```python
from build123d import *

# Parameters (mm, degrees)
SKETCH_1_W                      = 10
SKETCH_1_H                      = 110
CUT_EXTRUDE_1_REACH             = 12
SKETCH_2_R                      = 8.2
CUT_EXTRUDE_1_DIRECTION_2_DEPTH = 5
SKETCH_3_R                      = 1.4
CUT_EXTRUDE_2_DEPTH             = 11.0000001
CUT_EXTRUDE_2_DEPTH_BACK        = 11.0000001
FILLET_1_R                      = 10
FILLET_2_R                      = 10


with BuildPart() as part:
    # Sketch 1 → Revolve 1 (revolve)
    with BuildSketch(Plane.XY):
        with Locations((5, 55)):
            Rectangle(SKETCH_1_W, SKETCH_1_H)
    revolve(axis=Axis((0, 0, 0), (0, 1, 0)))

    # Sketch 2 → Cut-Extrude 1 (cut, up to next)
    with BuildSketch(Plane.XY, mode=Mode.PRIVATE) as cut_extrude_1_sk1:
        with Locations((0, 30)):
            Circle(SKETCH_2_R)
    cut_extrude_1_tool1 = extrude(cut_extrude_1_sk1.sketch, amount=-CUT_EXTRUDE_1_REACH, mode=Mode.PRIVATE) & part.part
    add(cut_extrude_1_tool1.solids().sort_by_distance((0, 30, 0))[0], mode=Mode.SUBTRACT)

    # Sketch 2 → Cut-Extrude 1 direction 2 (cut)
    with BuildSketch(Plane.XY):
        with Locations((0, 30)):
            Circle(SKETCH_2_R)
    extrude(amount=CUT_EXTRUDE_1_DIRECTION_2_DEPTH, mode=Mode.SUBTRACT)

    # Sketch 3 → Cut-Extrude 2 (cut, two sides)
    with BuildSketch(Plane(origin=(0, 0, 0), x_dir=(0, 0, -1), z_dir=(1, 0, 0))) as cut_extrude_2_sk:
        with Locations((0, 30)):
            Circle(SKETCH_3_R)
    extrude(amount=CUT_EXTRUDE_2_DEPTH, mode=Mode.SUBTRACT)
    extrude(cut_extrude_2_sk.sketch, amount=-CUT_EXTRUDE_2_DEPTH_BACK, mode=Mode.SUBTRACT)

    # Fillet 1
    fillet_1_edges = [part.edges().sort_by_distance(p)[0] for p in [
        (-10, 0, 0),
    ]]
    fillet(fillet_1_edges, radius=FILLET_1_R)

    # Fillet 2
    fillet_2_edges = [part.edges().sort_by_distance(p)[0] for p in [
        (-10, 110, 0),
    ]]
    fillet(fillet_2_edges, radius=FILLET_2_R)


solid = part.part
```
Source: CAD feature listing. Evaluate the final solid. Frame: model axes, mm. Coordinates: 2 decimals unless noted, no trailing zeros. Write each loop counter-clockwise with the first axis right and the second up, starting at its lowest first coordinate (ties: lowest second). Pieces come first, ordered by that corner, then holes. Notation, with made-up numbers: (25.25, 14.5) -> (33.25, 14.5) arc R12 cw to (33.25, 26.5) -> close; hole circle Ø1 at (56, 55.25). An arc over 180 degrees is marked (long way). Return JSON: item names as keys, results as strings. Group by question number.
1) Ray query, line 1 along X through (y, z) = (37, -8.75); line 2 along Y through (x, z) = (0, -1.5); line 3 along Y through (x, z) = (0, -4). Return the intervals inside material, ascending.
2) Section query A-A, the plane z = 0. Return loops of the section in (x, y).
3) Contact query for flat-ended pins moving along their axis: P1, Ø4, axis at x = 6, y = 24, coming from the -Z side; P2, Ø4, axis at y = 12, z = 6.5, coming from the +X side; P3, Ø5, axis at x = 2.5, y = 28, coming from the -Z side. Output: stop coordinate, or through.
4) Mould query, pull axis Z, two halves, no side actions, for faces 1 (the face through (0, 30, 5)), 2 (the face through (-9.03, 30.06, 1.4)), 3 (the face through (-2.17, 55.63, 9.76)), 4 (the face through (9.03, 30.06, 1.4)). Classes: +Z half, -Z half, draft (parallel to the pull), parting line (faces both ways), or undercut.
5) Section query C-C, the plane y = 30. Return loops of the section in (x, z), plus the area to 3 significant figures.
6) Section query B-B, the plane x = 0. Return loops of the section in (y, z).
7) Section query D-D, the plane z = 8. Return loops of the section in (x, y).
From the geometry:
{
 "1": {"line 1": "-4.84 to -4.27, 4.27 to 4.84", "line 2": "0.11 to 21.8, 38.2 to 109.89", "line 3": "0.83 to 21.8, 38.2 to 109.17"},
 "2": {"outline": "(-10, 10) arc R10 ccw to (10, 10) -> (10, 28.6) -> (8.08, 28.6) arc R8.2 cw to (-8.08, 28.6) -> (-10, 28.6) -> close; (-10, 31.4) -> (-8.08, 31.4) arc R8.2 cw to (8.08, 31.4) -> (10, 31.4) -> (10, 100) arc R10 ccw to (-10, 100) -> close"},
 "3": {"P1": "z = -9.04", "P2": "x = 8.93", "P3": "z = 5"},
 "4": {"face 1": "-Z half", "face 2": "undercut", "face 3": "parting line", "face 4": "undercut"},
 "5": {"outline": "(-9.9, -1.4) arc R10 ccw to (-8.2, -5.72) -> (-8.2, -1.4) -> close; (-9.9, 1.4) -> (-8.2, 1.4) -> (-8.2, 5) -> (8.2, 5) -> (8.2, 1.4) -> (9.9, 1.4) arc R10 ccw to start; (8.2, -5.72) arc R10 ccw to (9.9, -1.4) -> (8.2, -1.4) -> close", "area": "79.2 mm²"},
 "6": {"outline": "(10, -10) -> (21.8, -10) -> (21.8, 5) -> (38.2, 5) -> (38.2, -10) -> (100, -10) arc R10 ccw to (100, 10) -> (10, 10) arc R10 ccw to start"},
 "7": {"outline": "(-6, 10) arc R6 ccw to (6, 10) -> (6, 100) arc R6 ccw to (-6, 100) -> close"}
}
